Here's the drawing with two shaded views (mm, measured from the low corner). I have some questions. A direction names the side the tool comes from. Give positions to 0.01 mm unless a question says otherwise; leave off trailing zeros. Loops run counter-clockwise (first coordinate to the right, second up) from the corner with the lowest first, then second, coordinate; pieces in that order, holes last. Notation, with made-up numbers: M -3,38 L 10,38 A11 ccw 10,57 Z; hole C 66,62.5 d4. An arc over 180 degrees is marked long. Write item = value, one per line. Start each with the question number.
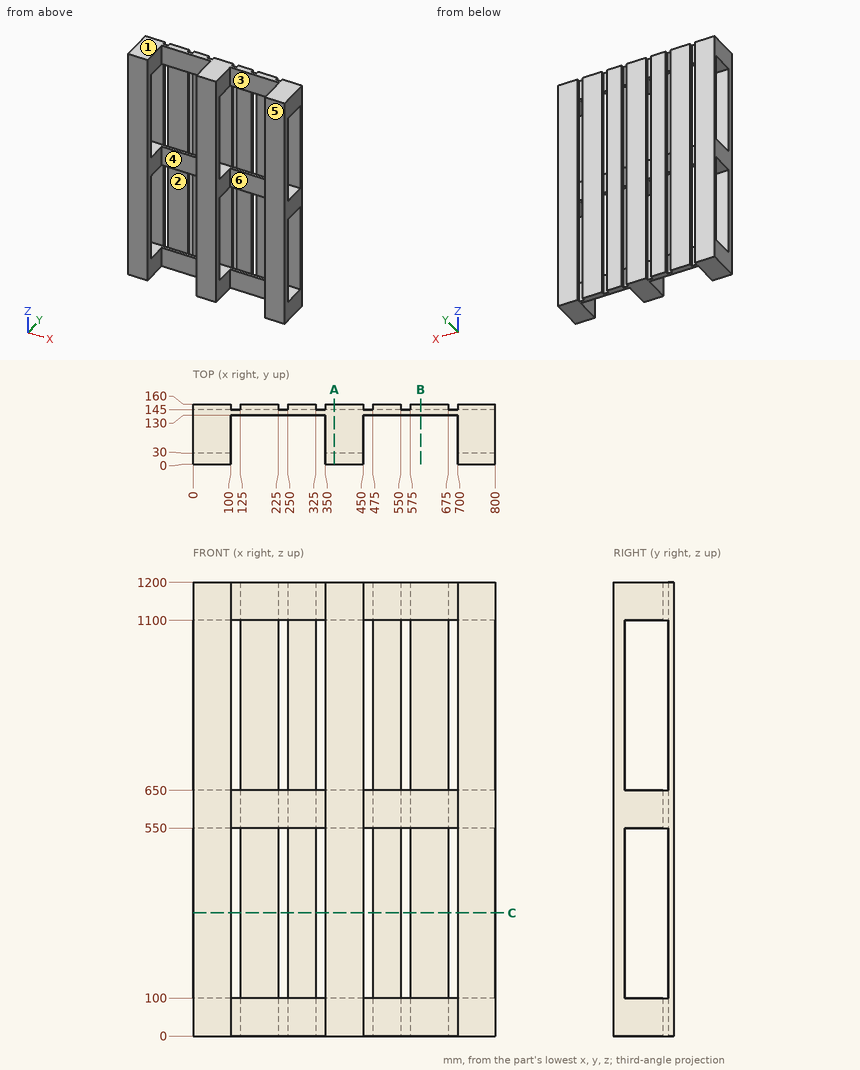
Q1. On a 3-axis mill with a long thin cutter (end or side, diameter ignored), from which of +Z, -Z, +X, -X, +Y, -Y can I reach the whole of each face in a straight line? I mean the marked faces 1, 2 and 3. Say none if no direction works.
Q2. We'd pull the mould along X, two halves only. Please class the marked faces 4, 5 and 6: pulls with the +X half, pulls with the -X half, needs draft (parallel to the pull), parting line crosses it, or undercut.
Q3. If we section it at B-B, the plane x = 602: List the corners of the cut face in (y, z) for me.
Q4. Will these pins go through, and if not, where does the flat tip stop? pin 1 (7.5 mm diameter, centred on y = 155.5, z = 513, fed in from -X); pin 2 (20 mm diameter, centred on x = 460.5, z = 52, fed in from +Y); pin 3 (1 mm diameter, centred on x = 542, z = 277.5, fed in from -Y).
Q5. If we section it at C-C, the plane z = 325.5: State how many separate pieces and enclosed holes the cut face has, then the cut area to 4 significant figures.
Q6. If we section it at A-A, the plane x = 373.5: List the corners of the cut face in (y, z) for me, then the cut area to 3 significant figures.
Q7. If I drill on line 1 along Z through (x, y) = (767.5, 74); line 2 along X through (y, z) = (58, 1137); line 3 along Y through (x, z) = (734, 125.5), over which ranges is the centre line in solid material (lowest first)?
Resolved:
q1.face_1 = +Z, +X, -X, +Y, -Y
q1.face_2 = +X, -X, -Y
q1.face_3 = +Z, -Z, -Y
q2.face_4 = undercut
q2.face_5 = needs draft
q2.face_6 = undercut
q3.outline = M 130,0 L 160,0 L 160,1200 L 130,1200 L 130,1100 L 145,1100 L 145,650 L 130,650 L 130,550 L 145,550 L 145,100 L 130,100 Z
q4.pin_1 = 0
q4.pin_2 = 145
q4.pin_3 = 145
q5.separate_pieces = 10
q5.enclosed_holes = 0
q5.area = 18,750 mm²
q6.outline = M 0,0 L 160,0 L 160,1200 L 0,1200 Z; hole M 30,100 L 145,100 L 145,550 L 30,550 Z; hole M 30,650 L 145,650 L 145,1100 L 30,1100 Z
q6.area = 88,500 mm²
q7.line_1 = 0 to 100, 550 to 650, 1100 to 1200
q7.line_2 = 0 to 100, 350 to 450, 700 to 800
q7.line_3 = 0 to 30, 145 to 160
